Check sheet for the modelled part. Datum: model origin and axes. Units: mm. Coordinates: 2 decimals unless noted, no trailing zeros. Loops run counter-clockwise (first coordinate to the right, second up) from the corner with the lowest first, then second, coordinate; pieces in that order, holes last.
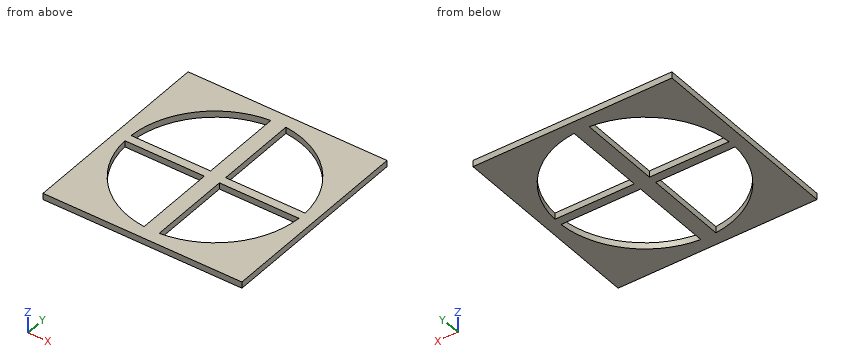
```python
from build123d import *

# Parameters (mm, degrees)
SKETCH1_W           = 80.01
SKETCH1_H           = 80.001
BOSS_EXTRUDE1_DEPTH = 5.08
SKETCH2_R           = 35.052
CUT_EXTRUDE1_DEPTH  = 5.08
SKETCH3_W           = 3.032686736
SKETCH3_H           = 3.433230268
BOSS_EXTRUDE3_DEPTH = 5.08
SKETCH5_W           = 135.597082566
SKETCH5_H           = 106.556051774
CUT_EXTRUDE2_DEPTH  = 2.54


with BuildPart() as part:
    # Sketch1 → Boss-Extrude1 (new body)
    with BuildSketch(Plane.XY):
        Rectangle(SKETCH1_W, SKETCH1_H)
    extrude(amount=BOSS_EXTRUDE1_DEPTH)

    # Sketch2 → Cut-Extrude1 (cut)
    with BuildSketch(Plane.XY.offset(5.08)):
        Circle(SKETCH2_R)
    extrude(amount=-CUT_EXTRUDE1_DEPTH, mode=Mode.SUBTRACT)

    # Sketch3 → Boss-Extrude3 (add)
    with BuildSketch(Plane.XY.offset(5.08)):
        with BuildLine():
            ThreePointArc((3.032686736, 34.920560064), (1.517766887, 35.019124599), (0, 35.052))
            Line((0, 35.052), (0, 1.716615134))
            Line((0, 1.716615134), (3.032686736, 1.716615134))
            Line((3.032686736, 1.716615134), (3.032686736, 34.920560064))
        make_face()
        with BuildLine():
            Line((0, 1.716615134), (0, 35.052))
            ThreePointArc((0, 35.052), (-1.517766887, 35.019124599), (-3.032686736, 34.920560064))
            Line((-3.032686736, 34.920560064), (-3.032686736, 1.716615134))
            Line((-3.032686736, 1.716615134), (0, 1.716615134))
        make_face()
        with BuildLine():
            Line((-3.032686736, -1.716615134), (-3.032686736, 1.716615134))
            Line((-3.032686736, 1.716615134), (-35.009940538, 1.716615134))
            ThreePointArc((-35.009940538, 1.716615134), (-35.052, 0), (-35.009940538, -1.716615134))
            Line((-35.009940538, -1.716615134), (-3.032686736, -1.716615134))
        make_face()
        with Locations((1.516343368, 0)):
            Rectangle(SKETCH3_W, SKETCH3_H)
        with Locations((-1.516343368, 0)):
            Rectangle(SKETCH3_W, SKETCH3_H)
        with BuildLine():
            Line((3.032686736, -1.716615134), (0, -1.716615134))
            Line((0, -1.716615134), (0, -35.052))
            ThreePointArc((0, -35.052), (1.517766887, -35.019124599), (3.032686736, -34.920560064))
            Line((3.032686736, -34.920560064), (3.032686736, -1.716615134))
        make_face()
        with BuildLine():
            Line((0, -35.052), (0, -1.716615134))
            Line((0, -1.716615134), (-3.032686736, -1.716615134))
            Line((-3.032686736, -1.716615134), (-3.032686736, -34.920560064))
            ThreePointArc((-3.032686736, -34.920560064), (-1.517766887, -35.019124599), (0, -35.052))
        make_face()
        with BuildLine():
            Line((35.009940538, 1.716615134), (3.032686736, 1.716615134))
            Line((3.032686736, 1.716615134), (3.032686736, -1.716615134))
            Line((3.032686736, -1.716615134), (35.009940538, -1.716615134))
            ThreePointArc((35.009940538, -1.716615134), (35.041483557, -0.858565157), (35.052, 0))
            ThreePointArc((35.052, 0), (35.041483557, 0.858565157), (35.009940538, 1.716615134))
        make_face()
    extrude(amount=-BOSS_EXTRUDE3_DEPTH)

    # Sketch5 → Cut-Extrude2 (cut)
    with BuildSketch(Plane.XY.offset(5.08)):
        with Locations((8.610263187, -0.677600572)):
            Rectangle(SKETCH5_W, SKETCH5_H)
    extrude(amount=-CUT_EXTRUDE2_DEPTH, mode=Mode.SUBTRACT)


solid = part.part
```
1) Section check B-B on y = -5. Enter the section's corners in (x, z) (3 decimals), plus the area to 3 significant figures.
Answer sheet:
outline: (-40.005, 0) - (-34.694, 0) - (-34.694, 2.54) - (-40.005, 2.54) - close; (-3.033, 0) - (3.033, 0) - (3.033, 2.54) - (-3.033, 2.54) - close; (34.694, 0) - (40.005, 0) - (40.005, 2.54) - (34.694, 2.54) - close
area: 42.4 mm2
2) Section check A-A on z = 1.1. Enter the section's corners in (x, y) (1 decimal), plus the area to 3 significant figures.
Answer sheet:
outline: (-40, -40) - (40, -40) - (40, 40) - (-40, 40) - close; hole (-35, -1.7) arc R35.1 ccw to (-3, -34.9) - (-3, -1.7) - close; hole (-35, 1.7) - (-3, 1.7) - (-3, 34.9) arc R35.1 ccw to start; hole (3, -34.9) arc R35.1 ccw to (35, -1.7) - (3, -1.7) - close; hole (3, 1.7) - (35, 1.7) arc R35.1 ccw to (3, 34.9) - close
area: 3,190 mm2
3) Section check C-C on x = -31. Enter the section's corners in (y, z), plus the area to 3 significant figures.
Answer sheet:
outline: (-40, 0) - (-16.36, 0) - (-16.36, 2.54) - (-40, 2.54) - close; (-1.72, 0) - (1.72, 0) - (1.72, 2.54) - (-1.72, 2.54) - close; (16.36, 0) - (40, 0) - (40, 2.54) - (16.36, 2.54) - close
area: 129 mm2
4) Scan lines: line 1 (Y direction, x = 28, z = 0.4); line 2 (X direction, y = -12, z = 0.15) (3 decimals); line 3 (Y direction, x = 19, z = 0.9). Record each from-to range of solid material in increasing order.
Answer sheet:
line 1: y = -40 to -21.09, -1.72 to 1.72, 21.09 to 40
line 2: x = -40.005 to -32.934, -3.033 to 3.033, 32.934 to 40.005
line 3: y = -40 to -29.46, -1.72 to 1.72, 29.46 to 40
5) Depth check by flat-ended pin: pin 1 (8 mm diameter, centred on x = -8.5, y = -17, fed in from +Z). Enter the tip coordinate at first touch or a pass-through.
Answer sheet:
pin 1: passes through
